Can you work these out from the model? Positions are in its coordinate system, mm. Give positions to 0.01 mm unless a question says otherwise; leave off trailing zeros. Loops run counter-clockwise (first coordinate to the right, second up) from the corner with the lowest first, then second, coordinate; pieces in that order, holes last. Notation, with made-up numbers: (34, 9) - (62, 9) arc R6 cw to (62, 17) - close; hole circle Ø6 at (57.25, -18.5). An arc over 180 degrees is marked (long way). Use a Markdown table: item, result. Add a question column.
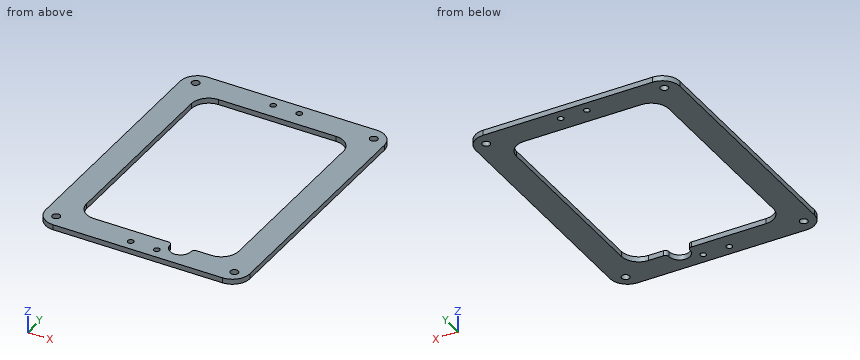
```python
from build123d import *

# Parameters (mm, degrees)
BOSS_EXTRU_1_START = 100
BOSS_EXTRU_1_DEPTH = 3
D_GAGEMENT_M41_D   = 4.5
CONG_1_R           = 2
D_GAGEMENT_M31_D   = 3.4


with BuildPart() as part:
    # Esquisse1 → Boss.-Extru.1 (new body)
    with BuildSketch(Plane.XY.offset(BOSS_EXTRU_1_START)):
        with BuildLine():
            ThreePointArc((-48.696481526, 0), (-55.767549338, -2.928932188), (-58.696481526, -10))
            Line((-58.696481526, -10), (-58.696481526, -145))
            ThreePointArc((-58.696481526, -145), (-55.767549338, -152.071067812), (-48.696481526, -155))
            Line((-48.696481526, -155), (48.696481526, -155))
            ThreePointArc((48.696481526, -155), (55.767549338, -152.071067812), (58.696481526, -145))
            Line((58.696481526, -145), (58.696481526, -10))
            ThreePointArc((58.696481526, -10), (55.767549338, -2.928932188), (48.696481526, 0))
            Line((48.696481526, 0), (-48.696481526, 0))
        make_face()
        with BuildLine():
            Line((-43.696481526, -130), (-43.696481526, -25))
            ThreePointArc((-43.696481526, -25), (-40.767549338, -17.928932188), (-33.696481526, -15))
            Line((-33.696481526, -15), (33.696481526, -15))
            ThreePointArc((33.696481526, -15), (40.767549338, -17.928932188), (43.696481526, -25))
            Line((43.696481526, -25), (43.696481526, -130))
            ThreePointArc((43.696481526, -130), (40.767549338, -137.071067812), (33.696481526, -140))
            Line((33.696481526, -140), (22.797478109, -140))
            ThreePointArc((22.797478109, -140), (23.07986531, -141.030472587), (23.175, -142.094693275))
            ThreePointArc((23.175, -142.094693275), (16.110779311, -147.999558585), (11.552521891, -140))
            Line((11.552521891, -140), (-33.696481526, -140))
            ThreePointArc((-33.696481526, -140), (-40.767549338, -137.071067812), (-43.696481526, -130))
        make_face(mode=Mode.SUBTRACT)
    extrude(amount=BOSS_EXTRU_1_DEPTH)

    # Dégagement M41 (through all)
    with Locations(Plane.XY.offset(103)):
        with Locations((-51.196481526, -7.5), (51.196481526, -7.5), (51.196481526, -147.5), (-51.196481526, -147.5)):
            Hole(D_GAGEMENT_M41_D / 2)

    # Congé1
    cong_1_edges = [part.edges().sort_by_distance(p)[0] for p in [
        (22.797478109, -140, 101.5),
        (11.552521891, -140, 101.5),
    ]]
    fillet(cong_1_edges, radius=CONG_1_R)

    # Dégagement M31 (through all)
    with Locations(Plane.XY.offset(103)):
        with Locations((-7.5, -6), (7.5, -6), (-7.5, -149), (7.5, -149)):
            Hole(D_GAGEMENT_M31_D / 2)


solid = part.part
```
1. Will this pin go through, and if not, where does the flat tip stop? P1, Ø2, axis at x = -7.5, y = -149, coming from the +Z side.
2. Suppose I cut it at B-B (x = 7.5). List the corners of the cut face in (y, z) for me, and give its area (3 significant figures).
3. Suppose I cut it at A-A (y = -109). List the corners of the cut face in (x, z) for me, and give its area (3 significant figures).
4. Suppose I cut it at D-D (z = 101.25). State how many separate pieces and enclosed holes the cut face has, and give its area (3 significant figures).
5. Suppose I cut it at C-C (x = 51). List the corners of the cut face in (y, z) for me, and give its area (3 significant figures).
6. Please list where these lines run through material, in increasing order: line 1 along Y through (x, z) = (-7.5, 101.6); line 2 along X through (y, z) = (-80.5, 101.9); line 3 along Y through (x, z) = (32, 101.2). Write a range as [from, to].
Results below:
| question | item | result |
|---|---|---|
| 1 | P1 | through |
| 2 | outline | (-155, 100) - (-150.7, 100) - (-150.7, 103) - (-155, 103) - close; (-147.3, 100) - (-140, 100) - (-140, 103) - (-147.3, 103) - close; (-15, 100) - (-7.7, 100) - (-7.7, 103) - (-15, 103) - close; (-4.3, 100) - (0, 100) - (0, 103) - (-4.3, 103) - close |
| 2 | area | 69.6 mm² |
| 3 | outline | (-58.7, 100) - (-43.7, 100) - (-43.7, 103) - (-58.7, 103) - close; (43.7, 100) - (58.7, 100) - (58.7, 103) - (43.7, 103) - close |
| 3 | area | 90.0 mm² |
| 4 | separate pieces | 1 |
| 4 | enclosed holes | 9 |
| 4 | area | 7,090 mm² |
| 5 | outline | (-154.73, 100) - (-149.74, 100) - (-149.74, 103) - (-154.73, 103) - close; (-145.26, 100) - (-9.74, 100) - (-9.74, 103) - (-145.26, 103) - close; (-5.26, 100) - (-0.27, 100) - (-0.27, 103) - (-5.26, 103) - close |
| 5 | area | 436 mm² |
| 6 | line 1 | [-155, -150.7], [-147.3, -140], [-15, -7.7], [-4.3, 0] |
| 6 | line 2 | [-58.7, -43.7], [43.7, 58.7] |
| 6 | line 3 | [-155, -140], [-15, 0] |
